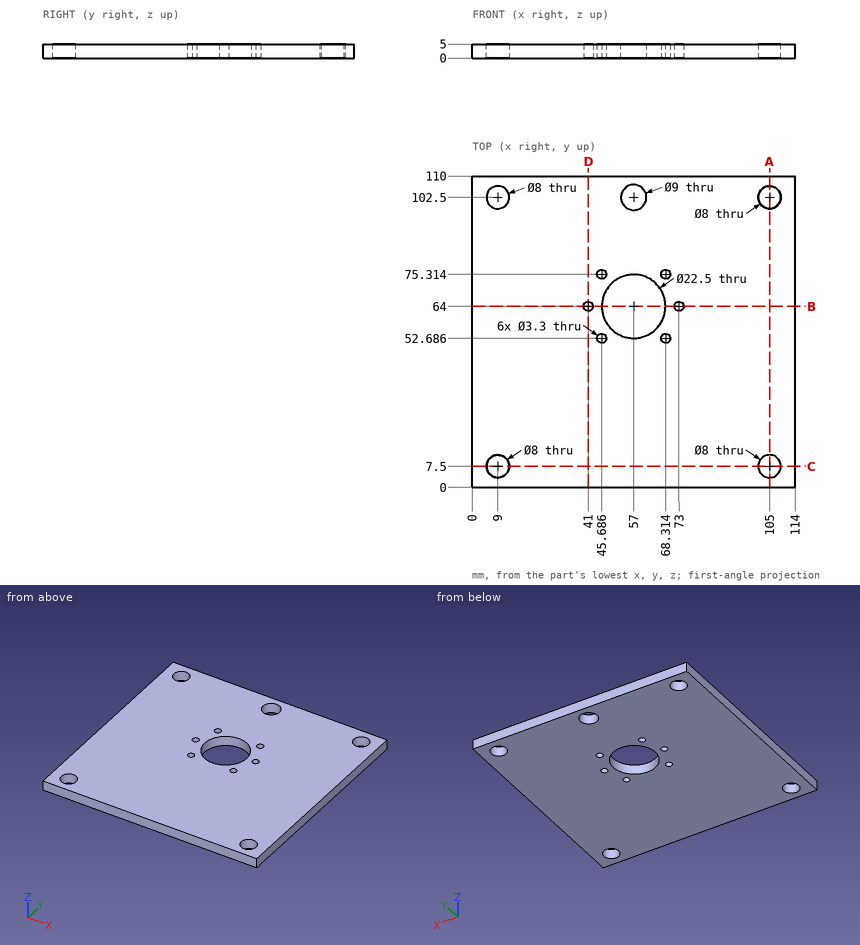
Drawing for the job (mm, zero at the part's lowest x, y, z). Round coordinates to 2 decimals unless told otherwise and drop trailing zeros. Loops run counter-clockwise (first coordinate to the right, second up) from the corner with the lowest first, then second, coordinate; pieces in that order, holes last. Notation, with made-up numbers: M 19,89.25 L 36,89.25 A30 ccw 36,121.25 Z; hole C 13.25,-29.5 d10. An arc over 180 degrees is marked long. Use a Markdown table: item, result. Add a question column.
(1) Cut at A-A (x = 105). Give the cut face in (y, z), and give its area (3 significant figures).
(2) Cut at D-D (x = 41). Give the cut face in (y, z).
(3) Drill centre lines: line 1 (Y direction, x = 9, z = 1.15); line 2 (X direction, y = 7.5, z = 1.85); line 3 (Y direction, x = 57, z = 1.2). Where is each one in solid material? Low to high.
(4) Cut at C-C (y = 7.5). Give the cut face in (x, z).
(5) Cut at B-B (y = 64). Give the cut face in (x, z).
Geometry says:
| question | item | result |
|---|---|---|
| 1 | outline | M 0,0 L 3.5,0 L 3.5,5 L 0,5 Z; M 11.5,0 L 98.5,0 L 98.5,5 L 11.5,5 Z; M 106.5,0 L 110,0 L 110,5 L 106.5,5 Z |
| 1 | area | 470 mm² |
| 2 | outline | M 0,0 L 62.35,0 L 62.35,5 L 0,5 Z; M 65.65,0 L 110,0 L 110,5 L 65.65,5 Z |
| 3 | line 1 | y = 0 to 3.5, 11.5 to 98.5, 106.5 to 110 |
| 3 | line 2 | x = 0 to 5, 13 to 101, 109 to 114 |
| 3 | line 3 | y = 0 to 52.75, 75.25 to 98, 107 to 110 |
| 4 | outline | M 0,0 L 5,0 L 5,5 L 0,5 Z; M 13,0 L 101,0 L 101,5 L 13,5 Z; M 109,0 L 114,0 L 114,5 L 109,5 Z |
| 5 | outline | M 0,0 L 39.35,0 L 39.35,5 L 0,5 Z; M 42.65,0 L 45.75,0 L 45.75,5 L 42.65,5 Z; M 68.25,0 L 71.35,0 L 71.35,5 L 68.25,5 Z; M 74.65,0 L 114,0 L 114,5 L 74.65,5 Z |
